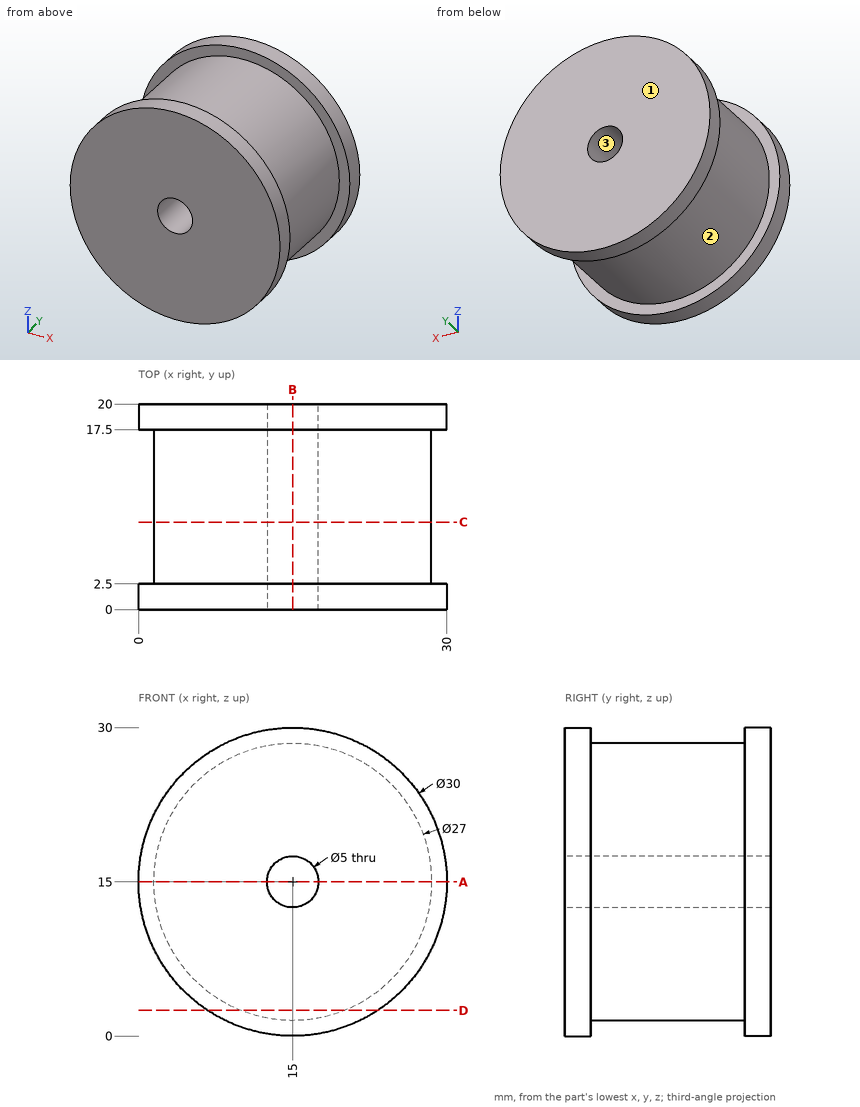
Here's the drawing with two shaded views (mm, measured from the low corner). I have some questions. Give positions to 0.01 mm unless a question says otherwise; leave off trailing zeros. Write each loop counter-clockwise with the first axis right and the second up, starting at its lowest first coordinate (ties: lowest second). Pieces come first, ordered by that corner, then holes. Notation, with made-up numbers: (5, -37.75) -> (24, -37.75) arc R9 ccw to (24, -26.75) -> close; hole circle Ø10 at (33.25, 47). An arc over 180 degrees is marked (long way). Answer as a JSON object with one key per item and string values. Group by question number.
Item 1: I'm going to push flat-ended pins straight in: P1, Ø5, axis at y = 13.5, z = 23.5, coming from the -X side; P2, Ø8, axis at x = 5.5, y = 13.5, coming from the -Z side; P3, Ø1.5, axis at y = 18, z = 13, coming from the +X side. Where does each tip first touch, or does it pass through?
Item 2: Suppose I cut it at B-B (x = 15). Please give me the cut outline in (y, z), plus the area to 3 significant figures.
Item 3: We'd pull the mould along Z, two halves only. Please class the marked faces 1, 2 and 3: +Z half, -Z half, draft (parallel to the pull), parting line (faces both ways), or undercut.
Item 4: Suppose I cut it at C-C (y = 8.5). Please give me the cut outline in (x, z).
Item 5: Please list where these lines run through material, in increasing order: line 1 (Y direction, x = 5.25, z = 4); line 2 (X direction, y = 11.5, z = 15). Write a range as [from, to].
Item 6: Suppose I cut it at A-A (z = 15). Please give me the cut outline in (x, y), plus the area to 3 significant figures.
Item 7: Suppose I cut it at D-D (z = 2.5). Please give me the cut outline in (x, y), plus the area to 3 significant figures.
Findings:
{
 "1": {"P1": "stops at x = 2.91", "P2": "stops at z = 2.67", "P3": "stops at x = 29.95"},
 "2": {"outline": "(0, 0) -> (2.5, 0) -> (2.5, 1.5) -> (17.5, 1.5) -> (17.5, 0) -> (20, 0) -> (20, 12.5) -> (0, 12.5) -> close; (0, 17.5) -> (20, 17.5) -> (20, 30) -> (17.5, 30) -> (17.5, 28.5) -> (2.5, 28.5) -> (2.5, 30) -> (0, 30) -> close", "area": "455 mm²"},
 "3": {"face 1": "draft", "face 2": "parting line", "face 3": "undercut"},
 "4": {"outline": "circle Ø27 at (15, 15); hole circle Ø5 at (15, 15)"},
 "5": {"line 1": "y = [0, 2.5], [17.5, 20]", "line 2": "x = [1.5, 12.5], [17.5, 28.5]"},
 "6": {"outline": "(0, 0) -> (12.5, 0) -> (12.5, 20) -> (0, 20) -> (0, 17.5) -> (1.5, 17.5) -> (1.5, 2.5) -> (0, 2.5) -> close; (17.5, 0) -> (30, 0) -> (30, 2.5) -> (28.5, 2.5) -> (28.5, 17.5) -> (30, 17.5) -> (30, 20) -> (17.5, 20) -> close", "area": "455 mm²"},
 "7": {"outline": "(6.71, 0) -> (23.29, 0) -> (23.29, 2.5) -> (20.1, 2.5) -> (20.1, 17.5) -> (23.29, 17.5) -> (23.29, 20) -> (6.71, 20) -> (6.71, 17.5) -> (9.9, 17.5) -> (9.9, 2.5) -> (6.71, 2.5) -> close", "area": "236 mm²"}
}
